```python
from build123d import *

# Parameters (mm, degrees)
F1_DEPTH = 70
F2_W     = 25.690172
F2_H     = 30
F3_DEPTH = 60
F6_DEPTH = 70.001


with BuildPart() as f1:
    # F0 (on Right) → F1 (new body, symmetric)
    with BuildSketch(Plane.YZ):
        with BuildLine():
            Line((10, 30), (0, 30))
            Line((0, 30), (0, 0))
            Line((0, 0), (-60, 0))
            Line((-60, 0), (-60, -30))
            Line((-60, -30), (-45, -30))
            ThreePointArc((-45, -30), (-25, -10), (-5, -30))
            Line((-5, -30), (0, -30))
            Line((0, -30), (10, -30))
            Line((10, -30), (10, 30))
        make_face()
    extrude(amount=F1_DEPTH, both=True)

    # F2 (on face) → F3 (join)
    with BuildSketch(Plane.XZ):
        with Locations((12.845086, 15)):
            Rectangle(F2_W, F2_H)
    extrude(amount=F3_DEPTH)

    # F4: F1 across plane


with BuildPart() as f1_1:
    add(f1.part)
    add(f1.part.mirror(Plane.YZ))

    # F5 (on face) → F6 (cut, through all)
    with BuildSketch(Plane.XZ.offset(60)):
        with BuildLine():
            Line((20, 30), (-20, 30))
            ThreePointArc((-20, 30), (0, 10), (20, 30))
        make_face()
    extrude(amount=-F6_DEPTH, mode=Mode.SUBTRACT)


solid = f1_1.part
```
For this review, take the finished solid that the model builds, in its own axes (mm). A direction names the side the tool comes from. Round coordinates to 2 decimals unless told otherwise and drop trailing zeros. Write each loop counter-clockwise with the first axis right and the second up, starting at its lowest first coordinate (ties: lowest second). Pieces come first, ordered by that corner, then holes. Notation, with made-up numbers: (-10, -22) -> (44, -22) arc R27 cw to (44, 16) -> close; hole circle Ø1 at (9.25, 23). An arc over 180 degrees is marked (long way). Use one line per item in the form item = value.
1) Clearance check with flat-ended pins moving along their axes: pin 1 (15 mm diameter, centred on y = -31, z = 15.5, fed in from +X); pin 2 (22 mm diameter, centred on x = 54, y = -21.5, fed in from +Z); pin 3 (9 mm diameter, centred on x = -53.5, z = 20, fed in from -Y); pin 4 (10 mm diameter, centred on x = 6.5, y = -43.5, fed in from -Z). State where each tip first meets the part, or that it passes through.
Found:
pin_1 = 25.69
pin_2 = 0
pin_3 = 0
pin_4 = -30
2) Take a section at A-A, the plane z = 5.5. Write out the cut boundary in (x, y).
Found:
outline = (-70, 0) -> (-25.69, 0) -> (-25.69, -60) -> (25.69, -60) -> (25.69, 0) -> (70, 0) -> (70, 10) -> (-70, 10) -> close
3) To check wall thickness, follow L1, parallel to X at y = -17, z = 8; L2, parallel to X at y = -28.5, z = 11.5; L3, parallel to Z at x = 58, y = -26. State the ranges of each line that lie inside material, in increasing order. Write a range as from..to.
Found:
L1 = -25.69..25.69
L2 = -25.69..-7.6, 7.6..25.69
L3 = -10.03..0
4) Take a section at C-C, the plane y = -41. Write out the cut boundary in (x, z), and give its area (3 significant figures).
Found:
outline = (-70, -18) -> (70, -18) -> (70, 0) -> (25.69, 0) -> (25.69, 30) -> (20, 30) arc R20 cw to (-20, 30) -> (-25.69, 30) -> (-25.69, 0) -> (-70, 0) -> close
area = 3,430 mm2
5) Take a section at D-D, the plane z = 24. Write out the cut boundary in (x, y).
Found:
outline = (-70, 0) -> (-25.69, 0) -> (-25.69, -60) -> (-19.08, -60) -> (-19.08, 10) -> (-70, 10) -> close; (19.08, -60) -> (25.69, -60) -> (25.69, 0) -> (70, 0) -> (70, 10) -> (19.08, 10) -> close
6) Take a section at B-B, the plane x = -44. Write out the cut boundary in (y, z).
Found:
outline = (-60, -30) -> (-45, -30) arc R20 cw to (-5, -30) -> (10, -30) -> (10, 30) -> (0, 30) -> (0, 0) -> (-60, 0) -> close
7) Mouldability with a two-part tool opening along Y and no side actions: class faces 4 (the flat face through (-48, -30, 0)), 5 (the flat face through (48, 0, 15)), 6 (the cylindrical face through (1, -25, -10)) as +Y half, -Y half, draft (parallel to the pull), parting line (faces both ways), or undercut.
Found:
face_4 = draft
face_5 = -Y half
face_6 = undercut
8) Tool access review of faces 1 (the cylindrical face through (0, -25, 10)), 2 (the flat face through (48, -30, 0)), 3 (the flat face through (-25.69, -30, 15)): name each direction out of +Z, -Z, +X, -X, +Y, -Y from which nothing blocks a thin tool from reaching the whole face with its end or side.
Found:
face_1 = +Z, +Y, -Y
face_2 = +Z, +X, -Y
face_3 = +Z, -X, -Y
